from build123d import *

# Parameters (mm, degrees)
SKETCH1_W           = 76.25
SKETCH1_H           = 76.25
SKETCH1_R           = 4
SKETCH1_W_2         = 56.25
SKETCH1_H_2         = 56.25
SKETCH1_R_2         = 1.6
BOSS_EXTRUDE1_DEPTH = 10
SKETCH2_R           = 3.5
CUT_EXTRUDE1_DEPTH  = 10
BOSS_EXTRUDE2_START = 10
SKETCH1_3_R         = 4
SKETCH1_3_R_2       = 1.6
BOSS_EXTRUDE2_DEPTH = 4


with BuildPart() as part:
    # Sketch1 → Boss-Extrude1 (new body)
    # profile 1 of 5: a face of its own
    with BuildSketch(Plane(origin=(0, 0, 0), x_dir=(1, 0, 0), z_dir=(0, 1, 0))):
        with Locations((28.125, -28.125)):
            Rectangle(SKETCH1_W, SKETCH1_H)
        with Locations((-5, 5)):
            Circle(SKETCH1_R, mode=Mode.SUBTRACT)
        with Locations((-5, -61.25)):
            Circle(SKETCH1_R, mode=Mode.SUBTRACT)
        with Locations((61.25, -61.25)):
            Circle(SKETCH1_R, mode=Mode.SUBTRACT)
        with Locations((61.25, 5)):
            Circle(SKETCH1_R, mode=Mode.SUBTRACT)
        with Locations((28.125, -28.125)):
            Rectangle(SKETCH1_W_2, SKETCH1_H_2, mode=Mode.SUBTRACT)
    # profile 2 of 5: a face of its own
    with BuildSketch(Plane(origin=(0, 0, 0), x_dir=(1, 0, 0), z_dir=(0, 1, 0))):
        with Locations((61.25, 5)):
            Circle(SKETCH1_R)
        with Locations(Location((61.25, 5, 0), (0, 0, 270))):
            Circle(SKETCH1_R_2, mode=Mode.SUBTRACT)
    # profile 3 of 5: a face of its own
    with BuildSketch(Plane(origin=(0, 0, 0), x_dir=(1, 0, 0), z_dir=(0, 1, 0))):
        with Locations((61.25, -61.25)):
            Circle(SKETCH1_R)
        with Locations(Location((61.25, -61.25, 0), (0, 0, 270))):
            Circle(SKETCH1_R_2, mode=Mode.SUBTRACT)
    # profile 4 of 5: a face of its own
    with BuildSketch(Plane(origin=(0, 0, 0), x_dir=(1, 0, 0), z_dir=(0, 1, 0))):
        with Locations((-5, -61.25)):
            Circle(SKETCH1_R)
        with Locations(Location((-5, -61.25, 0), (0, 0, 270))):
            Circle(SKETCH1_R_2, mode=Mode.SUBTRACT)
    # profile 5 of 5: a face of its own
    with BuildSketch(Plane(origin=(0, 0, 0), x_dir=(1, 0, 0), z_dir=(0, 1, 0))):
        with Locations((-5, 5)):
            Circle(SKETCH1_R)
        with Locations(Location((-5, 5, 0), (0, 0, 270))):
            Circle(SKETCH1_R_2, mode=Mode.SUBTRACT)
    extrude(amount=BOSS_EXTRUDE1_DEPTH)

    # Sketch2 → Cut-Extrude1 (cut)
    with BuildSketch(Plane(origin=(0, 0, 0), x_dir=(0, 0, -1), z_dir=(1, 0, 0))):
        with Locations((-28.125, 5)):
            Circle(SKETCH2_R)
    extrude(amount=-CUT_EXTRUDE1_DEPTH, mode=Mode.SUBTRACT)

    # Sketch1<3> → Boss-Extrude2 (add)
    # profile 1 of 4: a face of its own
    with BuildSketch(Plane(origin=(0, 0, 0), x_dir=(1, 0, 0), z_dir=(0, 1, 0)).offset(BOSS_EXTRUDE2_START)):
        with Locations(Location((-5, 5, 0), (0, 0, 270))):
            Circle(SKETCH1_3_R)
        with Locations(Location((-5, 5, 0), (0, 0, 270))):
            Circle(SKETCH1_3_R_2, mode=Mode.SUBTRACT)
    # profile 2 of 4: a face of its own
    with BuildSketch(Plane(origin=(0, 0, 0), x_dir=(1, 0, 0), z_dir=(0, 1, 0)).offset(BOSS_EXTRUDE2_START)):
        with Locations(Location((-5, -61.25, 0), (0, 0, 270))):
            Circle(SKETCH1_3_R)
        with Locations(Location((-5, -61.25, 0), (0, 0, 270))):
            Circle(SKETCH1_3_R_2, mode=Mode.SUBTRACT)
    # profile 3 of 4: a face of its own
    with BuildSketch(Plane(origin=(0, 0, 0), x_dir=(1, 0, 0), z_dir=(0, 1, 0)).offset(BOSS_EXTRUDE2_START)):
        with Locations(Location((61.25, -61.25, 0), (0, 0, 270))):
            Circle(SKETCH1_3_R)
        with Locations(Location((61.25, -61.25, 0), (0, 0, 270))):
            Circle(SKETCH1_3_R_2, mode=Mode.SUBTRACT)
    # profile 4 of 4: a face of its own
    with BuildSketch(Plane(origin=(0, 0, 0), x_dir=(1, 0, 0), z_dir=(0, 1, 0)).offset(BOSS_EXTRUDE2_START)):
        with Locations(Location((61.25, 5, 0), (0, 0, 270))):
            Circle(SKETCH1_3_R)
        with Locations(Location((61.25, 5, 0), (0, 0, 270))):
            Circle(SKETCH1_3_R_2, mode=Mode.SUBTRACT)
    extrude(amount=BOSS_EXTRUDE2_DEPTH)


solid = part.part
Part model, mm, in its own coordinate system. A direction names the side the tool comes from. Coordinates: 2 decimals unless noted, no trailing zeros. Order: outer loops, then holes, each group sorted by start corner. A loop starts at its lowest first (then second) coordinate and runs counter-clockwise, first axis right, second up. Notation, with made-up numbers: M 40.25,-23.75 L 76.25,-23.75 A22 cw 76.25,13.25 Z; hole C 39,-23.75 d5. An arc over 180 degrees is marked long. Use a Markdown table: item, result.
(1) Cut at B-B on x = -5. Write the cut outline in (y, z) (3 decimals), then the cut area to 3 significant figures.
A:
| item | result |
|---|---|
| outline | M 0,-10 L 10,-10 L 10,-9 L 14,-9 L 14,-6.6 L 0,-6.6 Z; M 0,-3.4 L 14,-3.4 L 14,-1 L 10,-1 L 10,57.25 L 14,57.25 L 14,59.65 L 0,59.65 Z; M 0,62.85 L 14,62.85 L 14,65.25 L 10,65.25 L 10,66.25 L 0,66.25 Z; hole C 5,28.125 d7 |
| area | 698 mm^2 |
(2) Flat gauge pins, fed straight in: pin 1 (23 mm diameter, centred on x = 11.5, z = 11, fed in from +Y); pin 2 (5.5 mm diameter, centred on y = 5, z = 28.125, fed in from -X). Where does each tip first touch, or does it go through?
A:
| item | result |
|---|---|
| pin 1 | stops at y = 10 |
| pin 2 | stops at x = 56.25 |
(3) Cut at C-C on y = 5. Write the cut outline in (x, z) (3 decimals), then the cut area to 3 significant figures.
A:
| item | result |
|---|---|
| outline | M -10,-10 L 66.25,-10 L 66.25,66.25 L -10,66.25 L -10,31.625 L 0,31.625 L 0,56.25 L 56.25,56.25 L 56.25,0 L 0,0 L 0,24.625 L -10,24.625 Z; hole C -5,-5 d3.2; hole C -5,61.25 d3.2; hole C 61.25,-5 d3.2; hole C 61.25,61.25 d3.2 |
| area | 2,550 mm^2 |
(4) Cut at D-D on z = 40. Write the cut outline in (x, y), then the cut area to 3 significant figures.
A:
| item | result |
|---|---|
| outline | M -10,0 L 0,0 L 0,10 L -10,10 Z; M 56.25,0 L 66.25,0 L 66.25,10 L 56.25,10 Z |
| area | 200 mm^2 |
(5) Probe L1, parallel to X at y = 6.5, z = 61.25; L2, parallel to Z at x = -3, y = 5.25; L3, parallel to Z at x = 62, y = 5.5. List the from-to ranges inside material, lowest first.
A:
| item | result |
|---|---|
| L1 | x = -10 to -6.6, -3.4 to 59.65, 62.85 to 66.25 |
| L2 | z = -10 to 24.63, 31.62 to 66.25 |
| L3 | z = -10 to -6.41, -3.59 to 59.84, 62.66 to 66.25 |
(6) Cut at A-A on z = -5. Write the cut outline in (x, y), then the cut area to 3 significant figures.
A:
| item | result |
|---|---|
| outline | M -10,0 L -6.6,0 L -6.6,14 L -9,14 L -9,10 L -10,10 Z; M -3.4,0 L 59.65,0 L 59.65,14 L 57.25,14 L 57.25,10 L -1,10 L -1,14 L -3.4,14 Z; M 62.85,0 L 66.25,0 L 66.25,10 L 65.25,10 L 65.25,14 L 62.85,14 Z |
| area | 737 mm^2 |
(7) Pull direction Z, two halves, no side cores. Call faces 1 (the cylindrical face through (-4.519, 6.902, 62.776)), 2 (the flat face through (-0.3, 0, 30.8)), 3 (the flat face through (28, 5, -10)): released by +Z, released by -Z, zero draft, split by the parting line, or undercut.
A:
| item | result |
|---|---|
| face 1 | undercut |
| face 2 | zero draft |
| face 3 | released by -Z |
(8) Tool access for faces 4 (the cylindrical face through (-4.93, 3.66, 24.89)), 5 (the flat face through (-0.3, 10, 27.9)), 6 (the flat face through (66.25, 5, 29)), 7 (the flat face through (28, 5, 56.25)), 8 (the flat face through (-7, 14, -5)): list every direction of +Z, -Z, +X, -X, +Y, -Y with a clear straight run to the whole face (end or side of a thin tool).
A:
| item | result |
|---|---|
| face 4 | -X |
| face 5 | +Y |
| face 6 | +Z, -Z, +X, +Y, -Y |
| face 7 | +Y, -Y |
| face 8 | +Z, -Z, +X, -X, +Y |
